CAD build for the part. Positions are in the model's coordinates, mm. Face numbers are marked on the shaded views. A direction names the side the tool comes from. Give positions to 0.01 mm unless a question says otherwise; leave off trailing zeros. Loops run counter-clockwise (first coordinate to the right, second up) from the corner with the lowest first, then second, coordinate; pieces in that order, holes last. Notation, with made-up numbers: M -6,75 L 2,75 A7 ccw 2,79 Z; hole C -12.5,-8 d7. An arc over 180 degrees is marked long. Answer as CSV lines item,"result".
from build123d import *

# Parameters (mm, degrees)
F0_R     = 32.084597
F1_DEPTH = 100
F2_R     = 10
F4_R     = 10.133801
F5_DEPTH = 125
F6_R     = 5


with BuildPart() as f1:
    # F0 (on Top) → F1 (new body)
    with BuildSketch(Plane.XY):
        Circle(F0_R)
    extrude(amount=F1_DEPTH)

    # F2
    f2_edges = [f1.edges().sort_by_distance(p)[0] for p in [
        (-32.084597, 0, 100),
        (-32.084597, 0, 0),
    ]]
    fillet(f2_edges, radius=F2_R)

    # F4 (on offset) → F5 (join)
    with BuildSketch(Plane.XZ.offset(26.2)):
        with Locations((0, 48.1227)):
            Circle(F4_R)
    extrude(amount=F5_DEPTH)

    # F6
    f6_edges = [f1.edges().sort_by_distance(p)[0] for p in [
        (-10.133801, -151.2, 48.1227),
    ]]
    fillet(f6_edges, radius=F6_R)


solid = f1.part
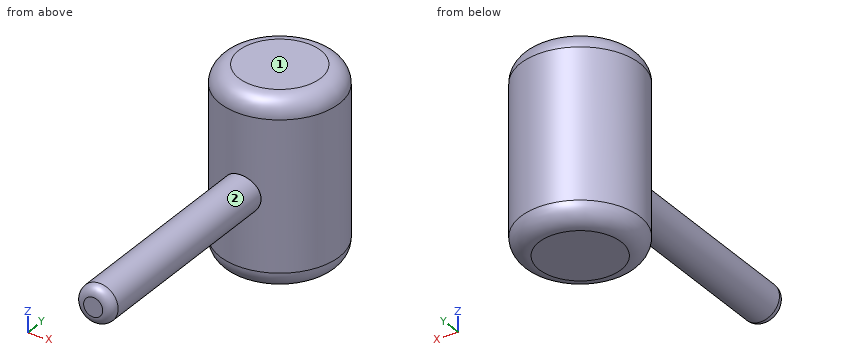
1) Which spindle directions (+Z, -Z, +X, -X, +Y, -Y) get a long thin tool onto all of the face, cutting with end or side? Do the marked faces 1 and 2. Say none if no direction does.
Answer below:
face 1,"+Z, +X, -X, +Y, -Y"
face 2,"-Y"
2) Band-saw the part on B-B on z = 62. Give the cut face in (x, y), and give its area (3 significant figures).
Answer below:
outline,"C 0,0 d64.17"
area,"3,230 mm^2"
3) Band-saw the part on C-C on y = -39.5. Give the cut face in (x, z), and give its area (3 significant figures).
Answer below:
outline,"C 0,48.12 d20.27"
area,"323 mm^2"
4) Band-saw the part on A-A on x = 0. Give the cut face in (y, z), and give its area (3 significant figures).
Answer below:
outline,"M -151.2,42.99 A5 ccw -146.2,37.99 L -32.08,37.99 L -32.08,10 A10 ccw -22.08,0 L 22.08,0 A10 ccw 32.08,10 L 32.08,90 A10 ccw 22.08,100 L -22.08,100 A10 ccw -32.08,90 L -32.08,58.26 L -146.2,58.26 A5 ccw -151.2,53.26 Z"
area,"8,730 mm^2"
5) Drill centre lines: line 1 (X direction, y = -1, z = 54.5); line 2 (X direction, y = -76, z = 48); line 3 (Y direction, x = 10.5, z = 52.5). Where is each one in solid material? Low to high. Write a range as from..to.
Answer below:
line 1,"x = -32.07..32.07"
line 2,"x = -10.13..10.13"
line 3,"y = -30.32..30.32"
6) Flat gauge pins, fed straight in: pin 1 (10 mm diameter, centred on y = -59.5, z = 36, fed in from -X); pin 2 (3 mm diameter, centred on y = -48, z = 50, fed in from -X); pin 3 (3 mm diameter, centred on x = 14.5, z = 58, fed in from -Y); pin 4 (8 mm diameter, centred on x = -15, y = -104, fed in from -Z). Where does each tip first touch, or does it go through?
Answer below:
pin 1,"stops at x = -7.21"
pin 2,"stops at x = -10.13"
pin 3,"stops at y = -29.33"
pin 4,"passes through"
